The listing builds one solid part. Answer for the finished solid, in the listing's coordinates (mm). Face numbers are marked on the shaded views. A direction names the side the tool comes from. Round coordinates to 2 decimals unless told otherwise and drop trailing zeros. Order: outer loops, then holes, each group sorted by start corner. A loop starts at its lowest first (then second) coordinate and runs counter-clockwise, first axis right, second up. Notation, with made-up numbers: (64, -13) - (109, -13) arc R29 cw to (109, 9) - close; hole circle Ø3 at (45.5, 74.5). An arc over 180 degrees is marked (long way). One line per item, written item: value. Start each with the question number.
1. Section A-A, the plane y = 19.05 is taken. Give the vertices of the cut face in (x, z) (3 decimals), then the cut area to 3 significant figures.
2. Section B-B, the plane z = 19 is taken. Give the vertices of the cut face in (x, y) (3 decimals).
3. A tool of negligible diameter and unlimited length cuts with its end or side. For the marked faces 1, 2, 3 and 4, from which of +Z, -Z, +X, -X, +Y, -Y can it reach the whole face along a straight path? Write none if from no direction.
4. Section D-D, the plane x = 59 is taken. Give the vertices of the cut face in (y, z).
5. Section C-C, the plane x = 35 is taken. Give the vertices of the cut face in (y, z), then the cut area to 3 significant figures.
6. Straight lines are drawn through the part: line 1 (Y direction, x = 38, z = 15); line 2 (X direction, y = 19, z = 16); line 3 (Z direction, x = 68.5, y = 7). For each, find the intervals that lie inside material, in ascending order.
7. Flat-ended cylindrical pins translate along their axes: P1, Ø5, axis at x = 62, y = 22, coming from the +Z side; P2, Ø3, axis at y = 14, z = 30, coming from the +X side; P3, Ø10, axis at y = 26.5, z = 32.5, coming from the -X side. Find the tip coordinate at first contact, or state that the pin passes through.
from build123d import *

# Parameters (mm, degrees)
F0_W          = 76.2
F0_H          = 38.1
F1_DEPTH      = 25.4
F2_R          = 19.05
F3_DEPTH      = 19.05
F3_DEPTH_BACK = 44.45
F4_R          = 9.525
F5_DEPTH      = 63.501


with BuildPart() as f1:
    # F0 (on Top) → F1 (new body)
    with BuildSketch(Plane.XY):
        with Locations((38.1, 19.05)):
            Rectangle(F0_W, F0_H)
    extrude(amount=F1_DEPTH)

    # F2 (on face) → F3 (join, two sides)
    with BuildSketch(Plane.XY.offset(25.4)) as f3_sk:
        with Locations((38.1, 19.05)):
            Circle(F2_R)
    extrude(amount=F3_DEPTH)
    extrude(f3_sk.sketch, amount=-F3_DEPTH_BACK)

    # F4 (on face) → F5 (cut, through all)
    with BuildSketch(Plane.XY.offset(44.45)):
        with Locations((38.1, 19.05)):
            Circle(F4_R)
    extrude(amount=-F5_DEPTH, mode=Mode.SUBTRACT)


solid = f1.part
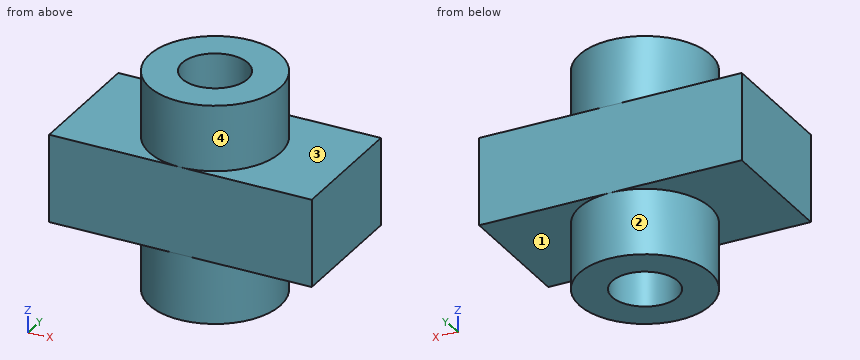
Answer list:
1. outline: (0, 0) - (19.05, 0) - (19.05, -19.05) - (28.575, -19.05) - (28.575, 44.45) - (19.05, 44.45) - (19.05, 25.4) - (0, 25.4) - close; (47.625, -19.05) - (57.15, -19.05) - (57.15, 0) - (76.2, 0) - (76.2, 25.4) - (57.15, 25.4) - (57.15, 44.45) - (47.625, 44.45) - close
1. area: 2,180 mm²
2. outline: (0, 0) - (76.2, 0) - (76.2, 38.1) - (0, 38.1) - close; hole circle Ø19.05 at (38.1, 19.05)
3. face 1: -Z, +X
3. face 2: -Z
3. face 3: +Z, +X
3. face 4: +Z
4. outline: (0, 0) - (38.1, 0) - (38.1, 25.4) - (0, 25.4) - close
5. outline: (0, 0) - (0.25, 0) - (0.25, -19.05) - (10.04, -19.05) - (10.04, 44.45) - (0.25, 44.45) - (0.25, 25.4) - (0, 25.4) - close; (28.06, -19.05) - (37.85, -19.05) - (37.85, 0) - (38.1, 0) - (38.1, 25.4) - (37.85, 25.4) - (37.85, 44.45) - (28.06, 44.45) - close
5. area: 1,260 mm²
6. line 1: y = 0 to 9.53, 28.57 to 38.1
6. line 2: x = 0 to 28.58, 47.62 to 76.2
6. line 3: z = 0 to 25.4
7. P1: stops at z = 25.4
7. P2: stops at x = 56.82
7. P3: stops at x = 19.21
